from build123d import *

# Parameters (mm, degrees)
SKETCH_1_W          = 56
SKETCH_1_H          = 25
SKETCH_1_R          = 3.5
EXTRUDE_1_DEPTH     = 3
CUT_EXTRUDE_1_DEPTH = 4
SKETCH_3_W          = 56
SKETCH_3_H          = 3
EXTRUDE_2_DEPTH     = 50
SKETCH_4_R          = 1.6
SKETCH_4_R_2        = 6.1
CUT_EXTRUDE_4_DEPTH = 40


with BuildPart() as part:
    # ｽｹｯﾁ1 → ﾎﾞｽ - 押し出し1 (new body)
    with BuildSketch(Plane.XY):
        Rectangle(SKETCH_1_W, SKETCH_1_H)
        with Locations((-18, 7)):
            Circle(SKETCH_1_R, mode=Mode.SUBTRACT)
        with Locations((18, 7)):
            Circle(SKETCH_1_R, mode=Mode.SUBTRACT)
    extrude(amount=EXTRUDE_1_DEPTH)

    # ｽｹｯﾁ2 → ｶｯﾄ - 押し出し1 (cut, through all)
    with BuildSketch(Plane.XY.offset(3)):
        with BuildLine():
            ThreePointArc((-21.4, 7.5), (-21.86862915, 8.63137085), (-23, 9.1))
            Line((-23, 9.1), (-23, 7.5))
            Line((-23, 7.5), (-24.6, 7.5))
            ThreePointArc((-24.6, 7.5), (-23, 5.9), (-21.4, 7.5))
        make_face()
        with BuildLine():
            Line((-23, 7.5), (-23, 9.1))
            ThreePointArc((-23, 9.1), (-24.13137085, 8.63137085), (-24.6, 7.5))
            Line((-24.6, 7.5), (-23, 7.5))
        make_face()
        with BuildLine():
            ThreePointArc((-24.6, -7.5), (-24.13137085, -8.63137085), (-23, -9.1))
            Line((-23, -9.1), (-23, -7.5))
            Line((-23, -7.5), (-24.6, -7.5))
        make_face()
        with BuildLine():
            Line((-23, -7.5), (-23, -9.1))
            ThreePointArc((-23, -9.1), (-21.86862915, -8.63137085), (-21.4, -7.5))
            ThreePointArc((-21.4, -7.5), (-23, -5.9), (-24.6, -7.5))
            Line((-24.6, -7.5), (-23, -7.5))
        make_face()
        with BuildLine():
            ThreePointArc((24.6, 7.5), (24.13137085, 8.63137085), (23, 9.1))
            Line((23, 9.1), (23, 7.5))
            Line((23, 7.5), (24.6, 7.5))
        make_face()
        with BuildLine():
            Line((23, 7.5), (23, 9.1))
            ThreePointArc((23, 9.1), (21.86862915, 6.36862915), (24.6, 7.5))
            Line((24.6, 7.5), (23, 7.5))
        make_face()
        with BuildLine():
            ThreePointArc((24.6, -7.5), (21.86862915, -6.36862915), (23, -9.1))
            Line((23, -9.1), (23, -7.5))
            Line((23, -7.5), (24.6, -7.5))
        make_face()
        with BuildLine():
            Line((23, -7.5), (23, -9.1))
            ThreePointArc((23, -9.1), (24.13137085, -8.63137085), (24.6, -7.5))
            Line((24.6, -7.5), (23, -7.5))
        make_face()
    extrude(amount=-CUT_EXTRUDE_1_DEPTH, mode=Mode.SUBTRACT)

    # ｽｹｯﾁ3 → ﾎﾞｽ - 押し出し2 (add)
    with BuildSketch(Plane(origin=(0, 12.5, 0), x_dir=(1, 0, 0), z_dir=(0, 1, 0))):
        with Locations((0, -1.5)):
            Rectangle(SKETCH_3_W, SKETCH_3_H)
    extrude(amount=EXTRUDE_2_DEPTH)

    # ｽｹｯﾁ4 → ｶｯﾄ - 押し出し4 (cut)
    with BuildSketch(Plane.XY):
        with Locations((-7.875, 57.13990011)):
            Circle(SKETCH_4_R)
        with Locations((7.875, 57.13990011)):
            Circle(SKETCH_4_R)
        with Locations((15.75, 43.5)):
            Circle(SKETCH_4_R)
        with Locations((7.875, 29.86009989)):
            Circle(SKETCH_4_R)
        with Locations((-7.875, 29.86009989)):
            Circle(SKETCH_4_R)
        with Locations((-15.75, 43.5)):
            Circle(SKETCH_4_R)
        with Locations((0, 50.5)):
            Circle(SKETCH_4_R_2)
    extrude(amount=CUT_EXTRUDE_4_DEPTH, mode=Mode.SUBTRACT)


solid = part.part
Design review of the part built by this model. Coordinates are the model's own, in mm. Round coordinates to 2 decimals unless told otherwise and drop trailing zeros. Write each loop counter-clockwise with the first axis right and the second up, starting at its lowest first coordinate (ties: lowest second). Pieces come first, ordered by that corner, then holes. Notation, with made-up numbers: (89, -16) -> (112, -16) arc R36 ccw to (112, 18) -> close; hole circle Ø1 at (78.5, -21.75). An arc over 180 degrees is marked (long way). One line per item, written item: value. Start each with the question number.
Q1. Add section C-C (z = 1.1). State how many separate pieces and enclosed holes the cut face has, then the cut area to 3 significant figures.
Q2. Add section B-B (x = -19). Give the boundary of the cut face in (y, z).
Q3. Add section A-A (y = 50.5). Give the boundary of the cut face in (x, z).
Q4. To check wall thickness, follow probe 1 along X at (y, z) = (-7.5, 1.1); probe 2 along Y at (x, z) = (0, 1); probe 3 along Y at (x, z) = (-16, 1.4). State the ranges of each line that lie inside material, in increasing order.
Q5. The part is to be moulded in two halves that separate along Y. For faces 1 (the face through (14.506, 6.8, 1.479)), 2 (the face through (-28, 24, 2)), 3 (the face through (0, 62.5, 1)), say which applies: pulls with the +Y half, pulls with the -Y half, needs draft (parallel to the pull), parting line crosses it, or undercut.
Q6. Insertion check: P1, Ø4, axis at x = 7.88, y = 29.86, coming from the +Z side. The pin has a flat end and moves straight along its axis. Give the tip position at first contact, or say it passes through.
Response:
1. separate pieces: 1
1. enclosed holes: 11
1. area: 3,930 mm^2
2. outline: (-12.5, 0) -> (3.65, 0) -> (3.65, 3) -> (-12.5, 3) -> close; (10.35, 0) -> (62.5, 0) -> (62.5, 3) -> (10.35, 3) -> close
3. outline: (-28, 0) -> (-6.1, 0) -> (-6.1, 3) -> (-28, 3) -> close; (6.1, 0) -> (28, 0) -> (28, 3) -> (6.1, 3) -> close
4. probe 1: x = -28 to -24.6, -21.4 to 21.4, 24.6 to 28
4. probe 2: y = -12.5 to 44.4, 56.6 to 62.5
4. probe 3: y = -12.5 to 4.13, 9.87 to 41.92, 45.08 to 62.5
5. face 1: undercut
5. face 2: needs draft
5. face 3: pulls with the +Y half
6. P1: stops at z = 3
